Design review of the part built by this model. Coordinates are the model's own, in mm. A direction names the side the tool comes from. Coordinates: 2 decimals unless noted, no trailing zeros. Loops run counter-clockwise (first coordinate to the right, second up) from the corner with the lowest first, then second, coordinate; pieces in that order, holes last. Notation, with made-up numbers: (-31.75, 27) - (15.25, 27) arc R24 cw to (15.25, 53) - close; hole circle Ø5 at (44.25, -16). An arc over 180 degrees is marked (long way). Answer in a Markdown table with one row per item. Add a question column.
(1) Clearance check with flat-ended pins moving along their axes: pin 1 (4 mm diameter, centred on x = 30, y = 5, fed in from -Z); pin 2 (1.2 mm diameter, centred on y = 4, z = 1, fed in from +X); pin 3 (2 mm diameter, centred on x = 4, y = 4, fed in from +Z). State where each tip first meets the part, or that it passes through.
(2) To check wall thickness, follow L1, parallel to X at y = 2.75, z = 0.7; L2, parallel to X at y = -4.25, z = 0.1; L3, parallel to Y at x = 13, z = 1.1. State the ranges of each line that lie inside material, in increasing order. Write a range as [from, to].
(3) We need section D-D, the plane z = -0.5. Write out the cut boundary in (x, y), plus the area to 3 significant figures.
(4) For faces 1 (the face through (28.907, 4, 0)), 2 (the face through (4, 4, -2)), 3 (the face through (-4, 4, 2)), list the 3-axis set-ups (+Z, -Z, +X, -X, +Y, -Y) from which the entire face can be reached by the end or side of a thin tool; tool diameter is ignored.
(5) We need section C-C, the plane x = -31. Write out the cut boundary in (y, z), plus the area to 3 significant figures.
(6) We need section A-A, the plane y = 0.75. Write out the cut boundary in (x, z), plus the area to 3 significant figures.
(7) We need section B-B, the plane y = -5.75. Write out the cut boundary in (x, z).
(8) The part is to be moulded in two halves that separate along Z. For faces 4 (the face through (31, 4, -1.963)), 5 (the face through (-32.5, 3.7, 0)), 6 (the face through (4, 7.5, 0)), say which applies: released by +Z, released by -Z, zero draft, split by the parting line, or undercut.
from build123d import *

# Parameters (mm, degrees)
F0_W     = 70
F0_H     = 5
F1_DEPTH = 20
F3_DEPTH = 2.501
F4_DEPTH = 2.501
F5_W     = 2.45
F5_H     = 4
F6_DEPTH = 7.5


with BuildPart() as f1:
    # F0 (on Front) → F1 (new body)
    with BuildSketch(Plane.XZ):
        Rectangle(F0_W, F0_H)
    extrude(amount=F1_DEPTH)

    # F2 (on Top) → F3 (cut, through all)
    with BuildSketch(Plane.XY):
        Polygon((2.5, 0), (0, 0), (-2.5, 0), (-2.5, -10), (2.5, -10), align=None)
    extrude(amount=-F3_DEPTH, mode=Mode.SUBTRACT)

    # F2 (on Top) → F4 (cut, through all)
    with BuildSketch(Plane.XY):
        Polygon((2.5, 0), (0, 0), (-2.5, 0), (-2.5, -10), (2.5, -10), align=None)
    extrude(amount=F4_DEPTH, mode=Mode.SUBTRACT)

    # F5 (on Front) → F6 (join)
    with BuildSketch(Plane.XZ):
        with BuildLine():
            Line((28.90652, -1.963228), (32.440649, -1.963228))
            ThreePointArc((32.440649, -1.963228), (32.5, -0.00059), (32.440721, 1.962049))
            Line((32.440721, 1.962049), (28.90652, 1.962049))
            Line((28.90652, 1.962049), (28.90652, -1.963228))
        make_face()
        with BuildLine():
            Line((-28.95826, 1.719714), (-32.454469, 1.719714))
            ThreePointArc((-32.454469, 1.719714), (-32.5, -0.000563), (-32.45441, -1.720838))
            Line((-32.45441, -1.720838), (-28.95826, -1.720838))
            Line((-28.95826, -1.720838), (-28.95826, 1.719714))
        make_face()
        with Locations((-3.725, 0)):
            Rectangle(F5_W, F5_H)
        with Locations((3.725, 0)):
            Rectangle(F5_W, F5_H)
    extrude(amount=-F6_DEPTH)


solid = f1.part
Responses:
| question | item | result |
|---|---|---|
| 1 | pin 1 | stops at z = -1.96 |
| 1 | pin 2 | stops at x = 32.5 |
| 1 | pin 3 | stops at z = 2 |
| 2 | L1 | x = [-32.49, -28.96], [-4.95, -2.5], [2.5, 4.95], [28.91, 32.49] |
| 2 | L2 | x = [-35, -2.5], [2.5, 35] |
| 2 | L3 | y = [-20, 0] |
| 3 | outline | (-35, -20) - (35, -20) - (35, 0) - (32.5, 0) - (32.5, 7.5) - (28.91, 7.5) - (28.91, 0) - (4.95, 0) - (4.95, 7.5) - (2.5, 7.5) - (2.5, -10) - (-2.5, -10) - (-2.5, 7.5) - (-4.95, 7.5) - (-4.95, 0) - (-28.96, 0) - (-28.96, 7.5) - (-32.5, 7.5) - (-32.5, 0) - (-35, 0) - close |
| 3 | area | 1,440 mm2 |
| 4 | face 1 | +Z, -Z, +Y |
| 4 | face 2 | -Z, +X, -X, +Y |
| 4 | face 3 | +Z, +X, -X, +Y |
| 5 | outline | (-20, -2.5) - (0, -2.5) - (0, -1.72) - (7.5, -1.72) - (7.5, 1.72) - (0, 1.72) - (0, 2.5) - (-20, 2.5) - close |
| 5 | area | 126 mm2 |
| 6 | outline | (-32.45, -1.72) - (-28.96, -1.72) - (-28.96, 1.72) - (-32.45, 1.72) arc R32.5 ccw to start; (-4.95, -2) - (-2.5, -2) - (-2.5, 2) - (-4.95, 2) - close; (2.5, -2) - (4.95, -2) - (4.95, 2) - (2.5, 2) - close; (28.91, -1.96) - (32.44, -1.96) arc R32.5 ccw to (32.44, 1.96) - (28.91, 1.96) - close |
| 6 | area | 45.8 mm2 |
| 7 | outline | (-35, -2.5) - (-2.5, -2.5) - (-2.5, 2.5) - (-35, 2.5) - close; (2.5, -2.5) - (35, -2.5) - (35, 2.5) - (2.5, 2.5) - close |
| 8 | face 4 | released by -Z |
| 8 | face 5 | split by the parting line |
| 8 | face 6 | zero draft |
